Input: part model. Units: mm. Frame: model coordinates. Give positions to 0.01 mm unless a question says otherwise; leave off trailing zeros. Loops run counter-clockwise (first coordinate to the right, second up) from the corner with the lowest first, then second, coordinate; pieces in that order, holes last. Notation, with made-up numbers: M 28.25,52 L 48.25,52 A22 cw 48.25,65 Z; hole C 55,-32 d4. An arc over 180 degrees is marked long. Use a Markdown table: item, result. Add a question column.
from build123d import *

# Parameters (mm, degrees)
SKETCH002_R     = 11
PAD001_DEPTH    = 20
SKETCH003_R     = 5.25
POCKET001_DEPTH = 20
FILLET005_R     = 0.5
FILLET006_R     = 0.5


with BuildPart() as part:
    # Sketch002 → Pad001 (new body)
    with BuildSketch(Plane.XY):
        with Locations((40, 0)):
            Circle(SKETCH002_R)
    extrude(amount=PAD001_DEPTH)

    # Sketch003 (on Face2 of Pad001) → Pocket001 (cut)
    with BuildSketch(Plane(origin=(0, 0, 0), x_dir=(1, 0, 0), z_dir=(0, 0, -1))):
        with Locations((40, 0)):
            Circle(SKETCH003_R)
    extrude(amount=-POCKET001_DEPTH, mode=Mode.SUBTRACT)

    # Fillet005
    fillet005_edges = [part.edges().sort_by_distance(p)[0] for p in [
        (34.75, 0, 20),
    ]]
    fillet(fillet005_edges, radius=FILLET005_R)

    # Fillet006
    fillet006_edges = [part.edges().sort_by_distance(p)[0] for p in [
        (34.75, 0, 0),
    ]]
    fillet(fillet006_edges, radius=FILLET006_R)


solid = part.part
1) Contact query for flat-ended pins moving along their axis: P1, Ø12, axis at x = 39, y = 5, coming from the +Z side; P2, Ø1.5, axis at x = 37, z = 16, coming from the -Y side; P3, Ø1, axis at y = 6.5, z = 7.5, coming from the -X side. Output: stop coordinate, or through.
2) Section query B-B, the plane y = 0. Return the cut outline in (x, z), and give its area (3 significant figures).
3) Ray query, line 1 (Y direction, x = 40, z = 14.25); line 2 (Y direction, x = 41.5, z = 18.5); line 3 (X direction, y = -2.5, z = 9.75). Return the intervals inside material, ascending. Write a range as [from, to].
4) Section query D-D, the plane x = 33.5. Return the cut outline in (y, z).
5) Pull-direction query (Y, two-part tool) for faces 1 (the cylindrical face through (36.13, -3.55, 9.87)), 2 (the cylindrical face through (50.161, -4.213, 9.86)), 3 (the flat face through (45, -5, 20)); classes: pulls with the +Y half, pulls with the -Y half, needs draft (parallel to the pull), parting line crosses it, or undercut.
6) Section query C-C, the plane z = 18.5. Return the cut outline in (x, y).
7) Section query A-A, the plane x = 40. Return the cut outline in (y, z).
Entries:
| question | item | result |
|---|---|---|
| 1 | P1 | stops at z = 20 |
| 1 | P2 | stops at y = -10.77 |
| 1 | P3 | stops at x = 30.78 |
| 2 | outline | M 29,0 L 34.25,0 A0.5 ccw 34.75,0.5 L 34.75,19.5 A0.5 ccw 34.25,20 L 29,20 Z; M 45.25,0.5 A0.5 ccw 45.75,0 L 51,0 L 51,20 L 45.75,20 A0.5 ccw 45.25,19.5 Z |
| 2 | area | 230 mm² |
| 3 | line 1 | y = [-11, -5.25], [5.25, 11] |
| 3 | line 2 | y = [-10.9, -5.03], [5.03, 10.9] |
| 3 | line 3 | x = [29.29, 35.38], [44.62, 50.71] |
| 4 | outline | M -8.87,0 L 8.87,0 L 8.87,20 L -8.87,20 Z |
| 5 | face 1 | undercut |
| 5 | face 2 | parting line crosses it |
| 5 | face 3 | needs draft |
| 6 | outline | C 40,0 d22; hole C 40,0 d10.5 |
| 7 | outline | M -11,0 L -5.75,0 A0.5 ccw -5.25,0.5 L -5.25,19.5 A0.5 ccw -5.75,20 L -11,20 Z; M 5.25,0.5 A0.5 ccw 5.75,0 L 11,0 L 11,20 L 5.75,20 A0.5 ccw 5.25,19.5 Z |
